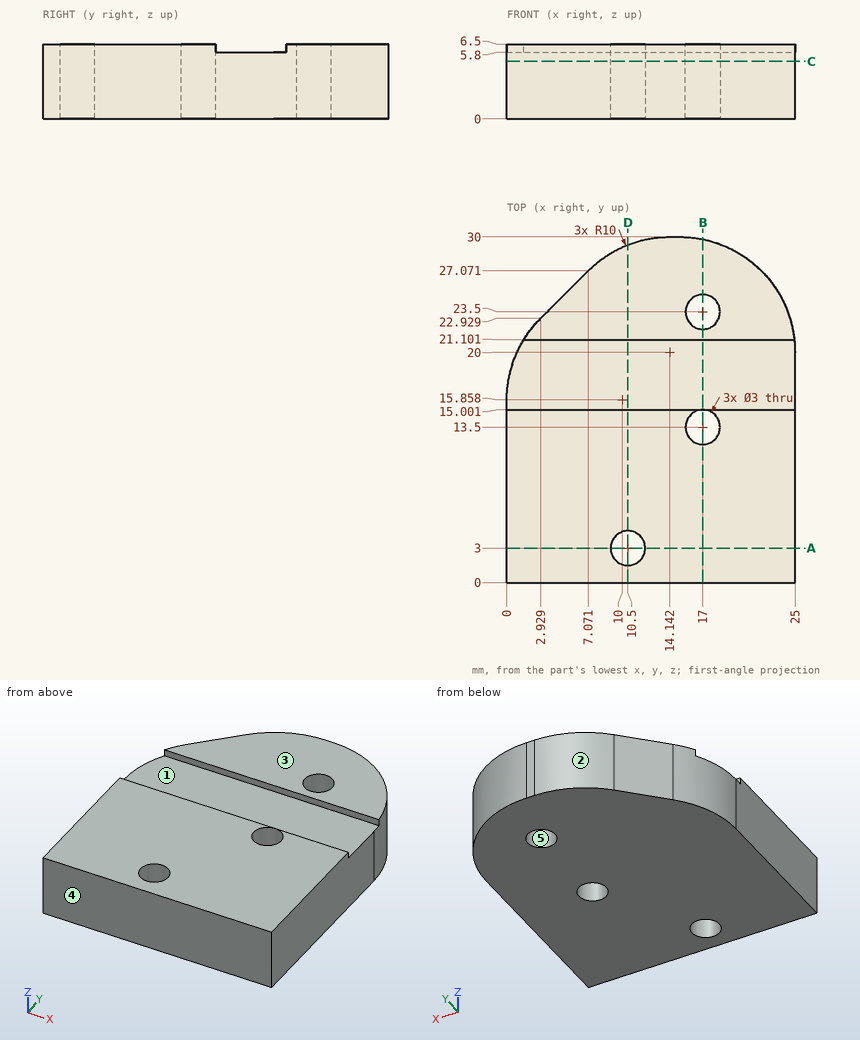
Answer from the drawing. Dimensions are ordinates in mm from the lowest x, y and z of the part. A direction names the side the tool comes from. Round coordinates to 2 decimals unless told otherwise and drop trailing zeros. Order: outer loops, then holes, each group sorted by start corner. A loop starts at its lowest first (then second) coordinate and runs counter-clockwise, first axis right, second up. Notation, with made-up numbers: (25.5, 15) - (29.5, 15) arc R11 ccw to (29.5, 29) - close; hole circle Ø6 at (-2.5, 89). An arc over 180 degrees is marked (long way). Put each result on its own line as item: value. Start each with the question number.
(1) For the marked faces 1 and 2, determine the directions among +Z, -Z, +X, -X, +Y, -Y from which every point of the face is accessible in a straight line to the end or side of a thin tool.
(2) Given P1, Ø3, axis at x = 12, y = 19, coming from the +Z side; P2, Ø0.6, axis at x = 17, z = 6, coming from the +Y side, each flat-ended and moving along its own axis, determine where each tip first touches the part or whether it passes through.
(3) Determine the mould class of the marked faces 3, 4 and 5 for opening direction Y: released by +Y, released by -Y, zero draft, split by the parting line, or undercut.
(4) Find section A-A (y = 3). Give the vertices of the cut face in (x, z).
(5) Straight lines are drawn through the part: probe 1 along Y at (x, z) = (17, 3.25); probe 2 along Z at (x, y) = (23.75, 16.75); probe 3 along Y at (x, z) = (9.25, 1.25). For each, find the intervals that lie inside material, in ascending order. Write a range as from..to.
(6) Find section B-B (x = 17). State how many separate pieces and enclosed holes the cut face has, plus the area to 3 significant figures.
(7) Find section D-D (x = 10.5). Give the vertices of the cut face in (y, z), plus the area to 3 significant figures.
(8) Find section C-C (z = 5). Give the vertices of the cut face in (x, y).
Reply:
1. face 1: +Z, +X, -X
1. face 2: +Z, -Z, -X, +Y
2. P1: z = 5.8
2. P2: y = 29.85
3. face 3: zero draft
3. face 4: released by -Y
3. face 5: undercut
4. outline: (0, 0) - (9, 0) - (9, 6.5) - (0, 6.5) - close; (12, 0) - (25, 0) - (25, 6.5) - (12, 6.5) - close
5. probe 1: 0..12, 15..22, 25..29.8
5. probe 2: 0..5.8
5. probe 3: 0..2.17, 3.83..28.72
6. separate pieces: 3
6. enclosed holes: 0
6. area: 150 mm^2
7. outline: (0, 0) - (1.5, 0) - (1.5, 6.5) - (0, 6.5) - close; (4.5, 0) - (29.31, 0) - (29.31, 6.5) - (21.1, 6.5) - (21.1, 5.8) - (15, 5.8) - (15, 6.5) - (4.5, 6.5) - close
7. area: 167 mm^2
8. outline: (0, 0) - (25, 0) - (25, 20) arc R10 ccw to (15, 30) - (14.14, 30) arc R10 ccw to (7.07, 27.07) - (2.93, 22.93) arc R10 ccw to (0, 15.86) - close; hole circle Ø3 at (10.5, 3); hole circle Ø3 at (17, 13.5); hole circle Ø3 at (17, 23.5)
